Input: part model. Units: mm. Frame: model coordinates. Coordinates: 2 decimals unless noted, no trailing zeros. Loops run counter-clockwise (first coordinate to the right, second up) from the corner with the lowest first, then second, coordinate; pieces in that order, holes last.
Item 1: Ray query, line 1 along Z through (x, y) = (26, 0); line 2 along X through (y, z) = (3.75, 0.15); line 3 along X through (y, z) = (-2.5, -0.2). Return the intervals inside material, ascending.
Item 2: Section A-A on y = 0. Return loops of the section in (x, z).
Item 3: Section B-B on x = 25. Return loops of the section in (y, z), and give its area (3 significant figures).
```python
from build123d import *

# Parameters (mm, degrees)
F2_R     = 0.5
F3_DEPTH = 4.5
F4_R     = 0.5
F5_DEPTH = 4.5


# Not quite as in the source:
# - a feature names something its author has since deleted; it is built from what else it names


with BuildPart() as f1:
    # F0 (on Top) → F1 (revolve)
    with BuildSketch(Plane.XY):
        with BuildLine():
            Line((44.3736289605, -1), (50.8157129178, -1.2541521454))
            ThreePointArc((50.8157129178, -1.2541521454), (50.4873850625, -0.6648939444), (50.3736289605, 0))
            Line((50.3736289605, 0), (-50.3736289605, 0))
            ThreePointArc((-50.3736289605, 0), (-50.4873850625, -0.6648939444), (-50.8157129178, -1.2541521454))
            Line((-50.8157129178, -1.2541521454), (-44.3736289605, -1))
            Line((-44.3736289605, -1), (44.3736289605, -1))
        make_face()
        with BuildLine():
            ThreePointArc((-50.8157129178, -1.2541521454), (-50.4873850625, -0.6648939444), (-50.3736289605, 0))
            Line((-50.3736289605, 0), (-51.8736289605, 0))
            Line((-51.8736289605, 0), (-52.8736289605, 0))
            Line((-52.8736289605, 0), (-54.3736289605, 0))
            ThreePointArc((-54.3736289605, 0), (-53.7878425229, -1.4142135624), (-52.3736289605, -2))
            ThreePointArc((-52.3736289605, -2), (-51.5100041261, -1.8039268681), (-50.8157129178, -1.2541521454))
        make_face()
        with BuildLine():
            ThreePointArc((52.3736289605, -2), (53.7878425229, -1.4142135624), (54.3736289605, 0))
            Line((54.3736289605, 0), (52.8736289605, 0))
            Line((52.8736289605, 0), (52.3736289605, 0))
            Line((52.3736289605, 0), (51.8736289605, 0))
            Line((51.8736289605, 0), (50.3736289605, 0))
            ThreePointArc((50.3736289605, 0), (50.4873850625, -0.6648939444), (50.8157129178, -1.2541521454))
            ThreePointArc((50.8157129178, -1.2541521454), (51.5100041261, -1.8039268681), (52.3736289605, -2))
        make_face()
    revolve(axis=Axis((0, 0, 0), (1, 0, 0)))

    # F2 (on Front) → F3 (join, symmetric)
    with BuildSketch(Plane.XZ):
        with Locations((-52.3736289605, 0)):
            Circle(F2_R)
    extrude(amount=F3_DEPTH, both=True)

    # F4 (on Front) → F5 (join, symmetric)
    with BuildSketch(Plane.XZ):
        with Locations((52.3736289605, 0)):
            Circle(F4_R)
    extrude(amount=F5_DEPTH, both=True)


solid = f1.part
```
Results found:
1. line 1: z = -1 to 1
1. line 2: x = -52.85 to -51.9, 51.9 to 52.85
1. line 3: x = -52.83 to -51.92, 51.92 to 52.83
2. outline: (-50.82, -1.25) - (-44.37, -1) - (44.37, -1) - (50.82, -1.25) arc R2 ccw (long way) to (50.82, 1.25) - (44.37, 1) - (-44.37, 1) - (-50.82, 1.25) arc R2 ccw (long way) to start
3. outline: circle Ø2 at (0, 0)
3. area: 3.14 mm2
